Work out the finished part from the listing and answer in its coordinate system (mm). A direction names the side the tool comes from. Coordinates: 2 decimals unless noted, no trailing zeros. Loops run counter-clockwise (first coordinate to the right, second up) from the corner with the lowest first, then second, coordinate; pieces in that order, holes last. Notation, with made-up numbers: (-23.5, 55) -> (23.5, 55) arc R30 ccw to (23.5, 89) -> close; hole circle Ø8 at (-3.75, 18). An arc over 180 degrees is marked (long way). One line per question, with ' | ' between items.
```python
from build123d import *

# Parameters (mm, degrees)
SKETCH1_W           = 22.225
SKETCH1_H           = 67.6402
BOSS_EXTRUDE1_DEPTH = 25.4
SKETCH2_R           = 1.7907
CUT_EXTRUDE2_DEPTH  = 25.4
SKETCH4_W           = 9.525
SKETCH4_H           = 10.16
SKETCH4_H_2         = 35.894850391
SKETCH4_H_3         = 35.916644849
CUT_EXTRUDE3_DEPTH  = 51.712797865
BOSS_EXTRUDE2_START = -43.154689
SKETCH5_R           = 2.38125
BOSS_EXTRUDE2_DEPTH = 57.632689


with BuildPart() as part:
    # Sketch1 → Boss-Extrude1 (new body)
    with BuildSketch(Plane.XY):
        with Locations((-17.147623967, 4.03062314)):
            Rectangle(SKETCH1_W, SKETCH1_H)
    extrude(amount=BOSS_EXTRUDE1_DEPTH)

    # Sketch2 → Cut-Extrude2 (cut)
    with BuildSketch(Plane.XY.offset(25.4)):
        with BuildLine():
            ThreePointArc((-20.309923967, 37.85072314), (-16.933347665, 36.452099442), (-15.534723967, 33.07552314))
            Line((-15.534723967, 33.07552314), (-15.534723967, 31.988846816))
            ThreePointArc((-15.534723967, 31.988846816), (-15.164047916, 28.377221194), (-14.067475414, 24.916185349))
            Line((-14.067475414, 24.916185349), (-13.85237252, 24.420060932))
            ThreePointArc((-13.85237252, 24.420060932), (-12.755800018, 20.959025087), (-12.385123967, 17.347399465))
            Line((-12.385123967, 17.347399465), (-12.385123967, 16.26072314))
            Line((-12.385123967, 16.26072314), (-6.035123967, 16.26072314))
            Line((-6.035123967, 16.26072314), (-6.035123967, 37.85072314))
            Line((-6.035123967, 37.85072314), (-20.309923967, 37.85072314))
        make_face()
        with BuildLine():
            Line((-25.085123967, 32.016111722), (-25.085123967, 33.07552314))
            ThreePointArc((-25.085123967, 33.07552314), (-23.686500268, 36.452099442), (-20.309923967, 37.85072314))
            Line((-20.309923967, 37.85072314), (-28.260123967, 37.85072314))
            Line((-28.260123967, 37.85072314), (-28.260123967, 17.320134559))
            ThreePointArc((-28.260123967, 17.320134559), (-27.884120973, 20.957343409), (-26.772015056, 24.440716329))
            Line((-26.772015056, 24.440716329), (-26.573232878, 24.895529952))
            ThreePointArc((-26.573232878, 24.895529952), (-25.461126961, 28.378902872), (-25.085123967, 32.016111722))
        make_face()
        with BuildLine():
            Line((-6.035123967, -29.78947686), (-6.035123967, 6.10072314))
            Line((-6.035123967, 6.10072314), (-12.385123967, 6.10072314))
            Line((-12.385123967, 6.10072314), (-12.385123967, -21.85197686))
            ThreePointArc((-12.385123967, -21.85197686), (-14.709963891, -27.464636935), (-20.322623967, -29.78947686))
            Line((-20.322623967, -29.78947686), (-6.035123967, -29.78947686))
        make_face()
        with BuildLine():
            ThreePointArc((-20.322623967, -29.78947686), (-25.935284043, -27.464636935), (-28.260123967, -21.85197686))
            Line((-28.260123967, -21.85197686), (-28.260123967, -29.78947686))
            Line((-28.260123967, -29.78947686), (-20.322623967, -29.78947686))
        make_face()
        with Locations((-20.309923967, 33.07552314)):
            Circle(SKETCH2_R)
    extrude(amount=-CUT_EXTRUDE2_DEPTH, mode=Mode.SUBTRACT)

    # Sketch4 → Cut-Extrude3 (cut, through all)
    with BuildSketch(Plane(origin=(-6.035123967, 0, 0), x_dir=(0, 0, -1), z_dir=(1, 0, 0))):
        with BuildLine():
            Line((-9.525, 16.698464592), (-9.525, 16.26072314))
            Line((-9.525, 16.26072314), (0, 16.26072314))
            Line((0, 16.26072314), (0, 32.637781689))
            ThreePointArc((0, 32.637781689), (-0.909409772, 28.750457477), (-3.448884978, 25.669973531))
            Line((-3.448884978, 25.669973531), (-6.076115022, 23.66627275))
            ThreePointArc((-6.076115022, 23.66627275), (-8.615590228, 20.585788804), (-9.525, 16.698464592))
        make_face()
        with Locations((-4.7625, 11.18072314)):
            Rectangle(SKETCH4_W, SKETCH4_H)
        with Locations((-4.7625, -11.846702056)):
            Rectangle(SKETCH4_W, SKETCH4_H_2)
        with Locations((-20.6375, -11.857599285)):
            Rectangle(SKETCH4_W, SKETCH4_H_3)
        with Locations((-20.6375, 11.18072314)):
            Rectangle(SKETCH4_W, SKETCH4_H)
        with BuildLine():
            Line((-25.4, 16.26072314), (-15.875, 16.26072314))
            Line((-15.875, 16.26072314), (-15.875, 16.698464592))
            ThreePointArc((-15.875, 16.698464592), (-16.784409772, 20.585788804), (-19.323884978, 23.66627275))
            Line((-19.323884978, 23.66627275), (-21.951115022, 25.669973531))
            ThreePointArc((-21.951115022, 25.669973531), (-24.490590228, 28.750457477), (-25.4, 32.637781689))
            Line((-25.4, 32.637781689), (-25.4, 16.26072314))
        make_face()
    extrude(amount=-CUT_EXTRUDE3_DEPTH, mode=Mode.SUBTRACT)

    # Sketch5 → Boss-Extrude2 (add)
    with BuildSketch(Plane(origin=(0, 0, 9.525), x_dir=(-1, 0, 0), z_dir=(0, 0, -1)).offset(BOSS_EXTRUDE2_START)):
        with Locations((20.322623967, -21.85197686)):
            Circle(SKETCH5_R)
    extrude(amount=BOSS_EXTRUDE2_DEPTH)


solid = part.part
```
1) Find section D-D (z = 39). Write down the section's boundary in (x, y), plus the area to 3 significant figures.
Check values:
outline: circle Ø4.76 at (-20.32, -21.85) | area: 17.8 mm^2
2) For faces 1 (the face through (-20.223, 24.682, 4.744)), 2 (the face through (-9, 16.261, 13)), 3 (the face through (-18.57, -20.24, 34.53)), determine the directions among +Z, -Z, +X, -X, +Y, -Y from which every point of the face is accessible in a straight line to the end or side of a thin tool.
Check values:
face 1: -Z, +X, -X | face 2: +Z, -Z, +X, +Y | face 3: +Z
3) Flat-ended cylindrical pins translate along their axes: pin 1 (8 mm diameter, centred on y = 25.5, z = 18.5, fed in from +X); pin 2 (4 mm diameter, centred on x = -19, y = 35.5, fed in from -Z); pin 3 (6 mm diameter, centred on x = -11, y = -13, fed in from -Z) (3 decimals). Find the tip coordinate at first contact, or state that the pin passes through.
Check values:
pin 1: stops at x = -12.91 | pin 2: stops at z = 0 | pin 3: stops at z = 9.525
4) Find section A-A (z = 13). Write down the section's boundary in (x, y) (1 decimal).
Check values:
outline: (-28.3, -21.9) arc R7.9 ccw to (-12.4, -21.9) -> (-12.4, 6.1) -> (-6, 6.1) -> (-6, 16.3) -> (-12.4, 16.3) -> (-12.4, 17.3) arc R17.8 ccw to (-13.9, 24.4) -> (-14.1, 24.9) arc R17.8 cw to (-15.5, 32) -> (-15.5, 33.1) arc R4.8 ccw to (-25.1, 33.1) -> (-25.1, 32) arc R17.8 cw to (-26.6, 24.9) -> (-26.8, 24.4) arc R17.8 ccw to (-28.3, 17.3) -> close; hole circle Ø3.6 at (-20.3, 33.1)
5) Find section B-B (x = -17). Write down the section's boundary in (y, z) (3 decimals), plus the area to 3 significant figures.
Check values:
outline: (-29.061, 9.525) -> (16.698, 9.525) arc R8.763 cw to (23.666, 6.076) -> (25.67, 3.449) arc R8.763 ccw to (32.638, 0) -> (36.517, 0) -> (36.517, 25.4) -> (32.638, 25.4) arc R8.763 ccw to (25.67, 21.951) -> (23.666, 19.324) arc R8.763 cw to (16.698, 15.875) -> (-29.061, 15.875) -> close | area: 642 mm^2
6) Find the intervals of material crossed by line 1 along Z through (x, y) = (-23.75, 16) (3 decimals); line 2 along Y through (x, z) = (-21, 20.5); line 3 along X through (y, z) = (-16, 12.5), in increasing order.
Check values:
line 1: z = 9.525 to 15.875 | line 2: y = -24.13 to -19.57, 24.56 to 31.42, 34.73 to 37.8 | line 3: x = -28.26 to -12.39
7) Find section C-C (y = -7). Write down the section's boundary in (x, z) (3 decimals), plus the area to 3 significant figures.
Check values:
outline: (-28.26, 9.525) -> (-12.385, 9.525) -> (-12.385, 15.875) -> (-28.26, 15.875) -> close | area: 101 mm^2
8) The mould has two halves that part along Y. Classify faces 4 (the face through (-20, 35, 0)), 5 (the face through (-18.57, -20.24, 2.39)), 6 (the face through (-25.47, 28.33, 12.88)), 7 (the face through (-20.232, 28.7, 24.465)): released by +Y, released by -Y, zero draft, split by the parting line, or undercut.
Check values:
face 4: zero draft | face 5: undercut | face 6: released by +Y | face 7: undercut
